The model under review builds one solid part; all positions refer to its coordinate system, in mm. A direction names the side the tool comes from. Coordinates: 2 decimals unless noted, no trailing zeros. Loops run counter-clockwise (first coordinate to the right, second up) from the corner with the lowest first, then second, coordinate; pieces in that order, holes last. Notation, with made-up numbers: M -1.75,-11 L 44.25,-11 A31 cw 44.25,21 Z; hole C -33.75,42 d10. An arc over 180 degrees is marked long. One line per item, written item: value.
```python
from build123d import *

# Parameters (mm, degrees)
SKETCH_1_W      = 80
SKETCH_1_H      = 45
SKETCH_1_R      = 10
SKETCH_1_W_2    = 2
SKETCH_1_H_2    = 20
EXTRUDE_1_DEPTH = 2


with BuildPart() as part:
    # Эскиз1 → Бобышка-Вытянуть1 (new body)
    # profile 1 of 3: a face of its own
    with BuildSketch(Plane.XY):
        with Locations((40, 22.5)):
            Rectangle(SKETCH_1_W, SKETCH_1_H)
        with Locations((40, 20)):
            Circle(SKETCH_1_R, mode=Mode.SUBTRACT)
    # profile 2 of 3: a face of its own
    with BuildSketch(Plane.XY):
        with Locations((81, 20)):
            Rectangle(SKETCH_1_W_2, SKETCH_1_H_2)
    # profile 3 of 3: a face of its own
    with BuildSketch(Plane.XY):
        with Locations((-1, 20)):
            Rectangle(SKETCH_1_W_2, SKETCH_1_H_2)
    extrude(amount=EXTRUDE_1_DEPTH)


solid = part.part
```
(1) Add section B-B on z = 0.35. State the section outline as (x, y) points, then the cut area to 3 significant figures.
Checks:
outline: M -2,10 L 0,10 L 0,0 L 80,0 L 80,10 L 82,10 L 82,30 L 80,30 L 80,45 L 0,45 L 0,30 L -2,30 Z; hole C 40,20 d20
area: 3,370 mm^2
(2) Draft analysis for pull direction X (two halves, no side actions). For faces 5 (the face through (0, 5, 1)), 6 (the face through (38.698, 29.915, 0.986)), 7 (the face through (30, 23, 2)), state which applies: pulls with the +X half, pulls with the -X half, needs draft (parallel to the pull), parting line crosses it, or undercut.
Checks:
face 5: pulls with the -X half
face 6: undercut
face 7: needs draft
(3) Insertion check: pin 1 Ø1 at (x, z) = (81, 0.5) entering from -Y; pin 2 Ø1 at (y, z) = (3.5, 1) entering from -X; pin 3 Ø0.6 at (x, z) = (-1, 0.5) entering from +Y. Each pin has a flat end and moves straight along its axis. Give the tip position at first contact, or say it passes through.
Checks:
pin 1: y = 10
pin 2: x = 0
pin 3: y = 30
(4) Tool access review of faces 1 (the face through (-1, 30, 1)), 2 (the face through (80, 5, 1)), 3 (the face through (-1, 10, 1)), 4 (the face through (81, 30, 1)): name each direction out of +Z, -Z, +X, -X, +Y, -Y from which nothing blocks a thin tool from reaching the whole face with its end or side.
Checks:
face 1: +Z, -Z, -X, +Y
face 2: +Z, -Z, +X, -Y
face 3: +Z, -Z, -X, -Y
face 4: +Z, -Z, +X, +Y
(5) Add section D-D on y = 39. State the section outline as (x, z) points.
Checks:
outline: M 0,0 L 80,0 L 80,2 L 0,2 Z
(6) To check wall thickness, follow L1, parallel to Y at x = 40, z = 1.35; L2, parallel to X at y = 30.5, z = 1.4; L3, parallel to Y at x = 47.5, z = 1.3. State the ranges of each line that lie inside material, in increasing order. Write a range as [from, to].
Checks:
L1: [0, 10], [30, 45]
L2: [0, 80]
L3: [0, 13.39], [26.61, 45]
(7) Add section A-A on x = 40. State the section outline as (y, z) points, then the cut area to 3 significant figures.
Checks:
outline: M 0,0 L 10,0 L 10,2 L 0,2 Z; M 30,0 L 45,0 L 45,2 L 30,2 Z
area: 50.0 mm^2
(8) Add section C-C on y = 20. State the section outline as (x, z) points.
Checks:
outline: M -2,0 L 30,0 L 30,2 L -2,2 Z; M 50,0 L 82,0 L 82,2 L 50,2 Z
